Design review of the part built by this model. Coordinates are the model's own, in mm. A direction names the side the tool comes from. Give positions to 0.01 mm unless a question says otherwise; leave off trailing zeros. Order: outer loops, then holes, each group sorted by start corner. A loop starts at its lowest first (then second) coordinate and runs counter-clockwise, first axis right, second up. Notation, with made-up numbers: (-7.5, 81) -> (29.5, 81) arc R28 cw to (29.5, 100) -> close; hole circle Ø5 at (67, 15). An arc over 180 degrees is marked (long way). Return JSON: item names as keys, results as strings.
```python
from build123d import *

# Parameters (mm, degrees)
SKETCH_1_W          = 100
SKETCH_1_H          = 52
EXTRUDE_1_DEPTH     = 8.6
SKETCH_2_W          = 97
SKETCH_2_H          = 49
CUT_EXTRUDE_1_DEPTH = 3
SKETCH_3_R          = 1.1
SKETCH_3_W          = 38.632034186
SKETCH_3_H          = 7.399361665
SKETCH_3_W_2        = 5
SKETCH_3_H_2        = 5
CUT_EXTRUDE_2_DEPTH = 61.603041755
FILLET_1_R          = 2
SKETCH_4_W          = 1.5
SKETCH_4_H          = 6.8
CUT_EXTRUDE_3_DEPTH = 1
SKETCH_5_W          = 97
SKETCH_5_H          = 49
CUT_EXTRUDE_4_DEPTH = 3
EXTRUDE_2_DEPTH     = 3
FILLET_2_R          = 3
FILLET_3_R          = 2
FILLET_5_R          = 1
SKETCH_9_W          = 52
SKETCH_9_H          = 4.3
CUT_EXTRUDE_5_DEPTH = 106.341399486


with BuildPart() as part:
    # 草图1 → 凸台-拉伸1 (new body)
    with BuildSketch(Plane(origin=(0, 0, 0), x_dir=(1, 0, 0), z_dir=(0, 1, 0))):
        with Locations((1.17145908, 5.982033169)):
            Rectangle(SKETCH_1_W, SKETCH_1_H)
    extrude(amount=EXTRUDE_1_DEPTH)

    # 草图2 → 切除-拉伸1 (cut)
    with BuildSketch(Plane.XZ):
        with Locations((1.17145908, -5.982033169)):
            Rectangle(SKETCH_2_W, SKETCH_2_H)
    extrude(amount=-CUT_EXTRUDE_1_DEPTH, mode=Mode.SUBTRACT)

    # 草图3 → 切除-拉伸2 (cut, through all)
    with BuildSketch(Plane.XZ.offset(-3)):
        with Locations(Location((-12.82854092, 15.517966831, 0), (0, 0, 270))):
            Circle(SKETCH_3_R)
        with Locations(Location((39.17145908, 15.517966831, 0), (0, 0, 270))):
            Circle(SKETCH_3_R)
        with Locations(Location((39.17145908, -27.482033169, 0), (0, 0, 270))):
            Circle(SKETCH_3_R)
        with Locations(Location((-12.82854092, -27.482033169, 0), (0, 0, 270))):
            Circle(SKETCH_3_R)
        with Locations((16.615396969, 13.018709543)):
            Rectangle(SKETCH_3_W, SKETCH_3_H)
        with Locations((-13.82854092, -12.482033169)):
            Rectangle(SKETCH_3_W_2, SKETCH_3_H_2)
        with Locations((23.17145908, -12.21289677)):
            Rectangle(SKETCH_3_W_2, SKETCH_3_H_2)
    extrude(amount=-CUT_EXTRUDE_2_DEPTH, mode=Mode.SUBTRACT)

    # 圆角1
    fillet_1_edges = [part.edges().sort_by_distance(p)[0] for p in [
        (20.67145908, 5.8, -14.71289677),
        (20.67145908, 5.8, -9.71289677),
        (25.67145908, 5.8, -9.71289677),
        (25.67145908, 5.8, -14.71289677),
        (-16.32854092, 5.8, -14.982033169),
        (-16.32854092, 5.8, -9.982033169),
        (-11.32854092, 5.8, -9.982033169),
        (-11.32854092, 5.8, -14.982033169),
    ]]
    fillet(fillet_1_edges, radius=FILLET_1_R)

    # 草图4 → 切除-拉伸3 (cut)
    with BuildSketch(Plane.XZ):
        with Locations((50.42145908, 0.917966831)):
            Rectangle(SKETCH_4_W, SKETCH_4_H)
    extrude(amount=-CUT_EXTRUDE_3_DEPTH, mode=Mode.SUBTRACT)

    # 草图5 → 切除-拉伸4 (cut)
    with BuildSketch(Plane(origin=(0, 8.6, 0), x_dir=(1, 0, 0), z_dir=(0, 1, 0))):
        with Locations((1.17145908, 5.982033169)):
            Rectangle(SKETCH_5_W, SKETCH_5_H)
    extrude(amount=-CUT_EXTRUDE_4_DEPTH, mode=Mode.SUBTRACT)

    # 草图7 → 凸台-拉伸2 (add, through all)
    with BuildSketch(Plane(origin=(0, 5.6, 0), x_dir=(1, 0, 0), z_dir=(0, 1, 0))):
        Polygon((-8.68854092, -18.517966831), (-8.68854092, 4.782033169), (-27.62854092, 4.782033169), (-27.62854092, 30.482033169), (-26.12854092, 30.482033169), (-26.12854092, 6.282033169), (-8.68854092, 6.282033169), (-8.68854092, 30.482033169), (-7.18854092, 30.482033169), (-7.18854092, -4.517966831), (49.67145908, -4.517966831), (49.67145908, -6.017966831), (-7.18854092, -6.017966831), (-7.18854092, -18.517966831), align=None)
        Polygon((16.97145908, 30.482033169), (16.97145908, 6.682033169), (30.17145908, 6.682033169), (30.17145908, 30.482033169), (28.67145908, 30.482033169), (28.67145908, 8.182033169), (18.47145908, 8.182033169), (18.47145908, 30.482033169), align=None)
    extrude(amount=EXTRUDE_2_DEPTH)

    # 圆角2
    fillet_2_edges = [part.edges().sort_by_distance(p)[0] for p in [
        (-48.82854092, 4.3, -31.982033169),
        (51.17145908, 4.3, -31.982033169),
        (51.17145908, 4.3, 20.017966831),
        (-48.82854092, 4.3, 20.017966831),
    ]]
    fillet(fillet_2_edges, radius=FILLET_2_R)

    # 圆角3
    fillet_3_edges = [part.edges().sort_by_distance(p)[0] for p in [
        (49.67145908, 1.5, 18.517966831),
        (49.67145908, 1.5, -30.482033169),
        (-47.32854092, 1.5, -30.482033169),
        (-47.32854092, 1.5, 18.517966831),
        (-47.32854092, 7.1, 18.517966831),
        (-47.32854092, 7.1, -30.482033169),
        (49.67145908, 7.1, -30.482033169),
        (49.67145908, 7.1, 18.517966831),
        (-8.68854092, 7.1, 18.517966831),
        (-7.18854092, 7.1, 18.517966831),
        (-7.18854092, 7.1, 6.017966831),
        (49.67145908, 7.1, 6.017966831),
        (49.67145908, 7.1, 4.517966831),
        (-7.18854092, 7.1, 4.517966831),
        (-7.18854092, 7.1, -30.482033169),
        (-8.68854092, 7.1, -30.482033169),
        (-8.68854092, 7.1, -6.282033169),
        (-26.12854092, 7.1, -6.282033169),
        (-26.12854092, 7.1, -30.482033169),
        (-27.62854092, 7.1, -30.482033169),
        (-27.62854092, 7.1, -4.782033169),
        (-8.68854092, 7.1, -4.782033169),
        (18.47145908, 7.1, -30.482033169),
        (16.97145908, 7.1, -30.482033169),
        (16.97145908, 7.1, -6.682033169),
        (30.17145908, 7.1, -6.682033169),
        (30.17145908, 7.1, -30.482033169),
        (28.67145908, 7.1, -30.482033169),
        (28.67145908, 7.1, -8.182033169),
        (18.47145908, 7.1, -8.182033169),
    ]]
    fillet(fillet_3_edges, radius=FILLET_3_R)

    # 圆角5
    fillet_5_edges = [part.edges().sort_by_distance(p)[0] for p in [
        (-2.700620124, 4.3, 16.718390375),
        (35.931414062, 4.3, 16.718390375),
        (-2.700620124, 4.3, 9.31902871),
        (35.931414062, 4.3, 9.31902871),
    ]]
    fillet(fillet_5_edges, radius=FILLET_5_R)

    # 草图9 → 切除-拉伸5 (cut, through all)
    with BuildSketch(Plane(origin=(51.17145908, 0, 0), x_dir=(0, 0, -1), z_dir=(1, 0, 0))):
        with Locations((5.982033169, 6.45)):
            Rectangle(SKETCH_9_W, SKETCH_9_H)
    extrude(amount=-CUT_EXTRUDE_5_DEPTH, mode=Mode.SUBTRACT)


solid = part.part
```
Item 1: Mouldability with a two-part tool opening along X and no side actions: class faces 1 (the face through (50.27, 2.18, 19.16)), 2 (the face through (40.262, 3.641, 15.661)), 3 (the face through (-11.738, 3.641, -27.339)), 4 (the face through (1, 0, -31)) as released by +X, released by -X, zero draft, split by the parting line, or undercut.
Result set:
{"face 1": "released by +X", "face 2": "undercut", "face 3": "undercut", "face 4": "zero draft"}
Item 2: Add section D-D (x = -8). Give the boundary of the cut face in (y, z), plus the area to 3 significant figures.
Result set:
{"outline": "(0, -31.98) -> (4.3, -31.98) -> (4.3, 20.02) -> (0, 20.02) -> (0, 18.52) -> (3, 18.52) -> (3, -30.48) -> (0, -30.48) -> close", "area": "76.6 mm^2"}
Item 3: Add section A-A (x = 16). Give the boundary of the cut face in (y, z).
Result set:
{"outline": "(0, -31.98) -> (4.3, -31.98) -> (4.3, 9.32) -> (3, 9.32) -> (3, -30.48) -> (0, -30.48) -> close; (0, 18.52) -> (3, 18.52) -> (3, 16.72) -> (4.3, 16.72) -> (4.3, 20.02) -> (0, 20.02) -> close"}
Item 4: Add section B-B (y = 2.05). Give the boundary of the cut face in (x, z), plus the area to 3 significant figures.
Result set:
{"outline": "(-48.83, -28.98) arc R3 ccw to (-45.83, -31.98) -> (48.17, -31.98) arc R3 ccw to (51.17, -28.98) -> (51.17, 17.02) arc R3 ccw to (48.17, 20.02) -> (-45.83, 20.02) arc R3 ccw to (-48.83, 17.02) -> close; hole (-47.33, -28.48) arc R2 ccw to (-45.33, -30.48) -> (47.67, -30.48) arc R2 ccw to (49.67, -28.48) -> (49.67, 16.52) arc R2 ccw to (47.67, 18.52) -> (-45.33, 18.52) arc R2 ccw to (-47.33, 16.52) -> close", "area": "443 mm^2"}
Item 5: For pin 1 (12 mm diameter, centred on x = -27.5, z = -10.5, fed in from -Y); pin 2 (0.5 mm diameter, centred on x = 50.5, y = 0.5, fed in from +Z), all flat-tipped, find the tip position at first contact; note any pin that passes through.
Result set:
{"pin 1": "stops at y = 3", "pin 2": "stops at z = 19.18"}
Item 6: Machinability: for faces 5 (the face through (-15.727, 3.659, -10.552)), 6 (the face through (0, 3, -6)), 7 (the face through (-47.97, 2.18, 19.12)), which of the approach directions +Z, -Z, +X, -X, +Y, -Y give a long, thin tool a straight path to every point of the face, cutting with its end or side? Answer none if there is none.
Result set:
{"face 5": "+Y, -Y", "face 6": "-Y", "face 7": "+Z, -X, +Y, -Y"}
Item 7: Wall thickness on L1, parallel to X at y = 3.45, z = -12; L2, parallel to Z at x = 21.5, y = 0.85; L3, parallel to X at y = 2.55, z = -21: over which ranges is each line inside the solid? List them lowest first. Write a range as [from, to].
Result set:
{"L1": "x = [-48.83, -16.33], [-11.33, 20.67], [25.67, 51.17]", "L2": "z = [-31.98, -30.48], [18.52, 20.02]", "L3": "x = [-48.83, -47.33], [49.67, 51.17]"}
Item 8: Add section C-C (z = -24). Give the boundary of the cut face in (x, y).
Result set:
{"outline": "(-48.83, 0) -> (-47.33, 0) -> (-47.33, 3) -> (49.67, 3) -> (49.67, 0) -> (51.17, 0) -> (51.17, 4.3) -> (-48.83, 4.3) -> close"}
